Part print with two shaded views. Sizes in mm from the minimum x, y, z corner. A direction names the side the tool comes from. Give positions to 0.01 mm unless a question says otherwise; leave off trailing zeros. Write each loop counter-clockwise with the first axis right and the second up, starting at its lowest first coordinate (ties: lowest second). Pieces come first, ordered by that corner, then holes.
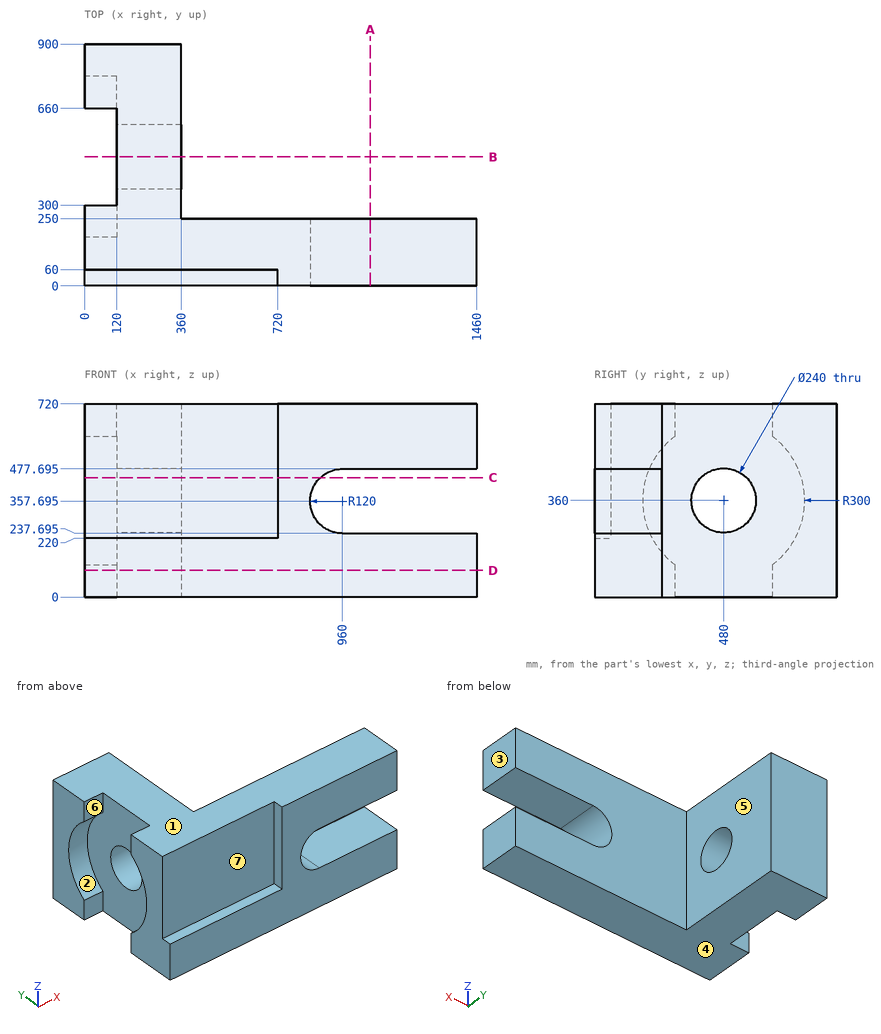
1) Drill centre lines: L1, parallel to Y at x = 255, z = 360; L2, parallel to Y at x = 1171.5, z = 217; L3, parallel to X at y = 42, z = 677. Where is each one in solid material? Low to high.
Check result:
L1: y = 60 to 360, 600 to 900
L2: y = 0 to 250
L3: x = 720 to 1460
2) Flat gauge pins, fed straight in: P1, Ø2, axis at y = 133, z = 268.5, coming from the +X side; P2, Ø6, axis at x = 511.5, z = 578, coming from the -Y side; P3, Ø1.5, axis at y = 150, z = 316.5, coming from the +X side. Where does each tip first touch, or does it go through?
Check result:
P1: stops at x = 880.85
P2: stops at y = 60
P3: stops at x = 847.57
3) Saw through at D-D (z = 100). Write the cut outline in (x, y), and give its area (3 significant figures).
Check result:
outline: (0, 0) - (1460, 0) - (1460, 250) - (360, 250) - (360, 900) - (0, 900) - (0, 660) - (120, 660) - (120, 300) - (0, 300) - close
area: 556,000 mm2
4) Saw through at A-A (x = 1064). Write the cut outline in (y, z) (1 decimal).
Check result:
outline: (0, 0) - (250, 0) - (250, 237.7) - (0, 237.7) - close; (0, 477.7) - (250, 477.7) - (250, 720) - (0, 720) - close
5) Saw through at C-C (z = 445.5). Write the cut outline in (x, y).
Check result:
outline: (0, 60) - (720, 60) - (720, 0) - (878.21, 0) - (878.21, 250) - (360, 250) - (360, 395.8) - (120, 395.8) - (120, 192.44) - (0, 192.44) - close; (0, 767.56) - (120, 767.56) - (120, 564.2) - (360, 564.2) - (360, 900) - (0, 900) - close
6) Saw through at B-B (y = 480). Write the cut outline in (x, z), and give its area (3 significant figures).
Check result:
outline: (120, 0) - (360, 0) - (360, 240) - (120, 240) - close; (120, 480) - (360, 480) - (360, 720) - (120, 720) - close
area: 115,000 mm2
7) Mould opens along Z. For the marked faces 1, 2, 3 and 4 say: +Z half, -Z half, draft (parallel to the pull), parting line (faces both ways), or undercut.
Check result:
face 1: +Z half
face 2: undercut
face 3: draft
face 4: -Z half
8) 3-axis set-ups, long thin cutter, end or side, ignore diameter. For the marked faces 5, 6 and 7: which of +Z, -Z, +X, -X, +Y, -Y reach the whole face in a straight line?
Check result:
face 5: +Z, -Z, +X, +Y
face 6: +Z, -Z, -X
face 7: +Z, -X, -Y
